Job drawing, mm, ordinate dimensions from the low corner. One solid piece. A direction names the side the tool comes from. Give positions to 0.01 mm unless a question says otherwise; leave off trailing zeros. Order: outer loops, then holes, each group sorted by start corner. A loop starts at its lowest first (then second) coordinate and runs counter-clockwise, first axis right, second up.
1. Which spindle directions (+Z, -Z, +X, -X, +Y, -Y) get a long thin tool onto all of the face, cutting with end or side? Do the marked faces 1, 2 and 3. Say none if no direction does.
2. Slice it at A-A on y = 12.7. List the corners of the cut face in (x, z), and give its area (3 significant figures).
3. Slice it at D-D on x = 190.5. List the corners of the cut face in (y, z).
4. Drop flat-ended pins along their axis: pin 1 Ø7.5 at (y, z) = (56, 10.5) entering from +X; pin 2 Ø10 at (x, z) = (234.5, 10) entering from +Y. Give the stop position or say it passes through.
5. Slice it at B-B on x = 279.4. List the corners of the cut face in (y, z).
6. Slice it at C-C on y = 63.5. List the corners of the cut face in (x, z).
7. Probe line 1 (Y direction, x = 114.3, z = 17.25); line 2 (X direction, y = 22, z = 11.5) (1 decimal); line 3 (X direction, y = 61, z = 5). List the from-to ranges inside material, lowest first.
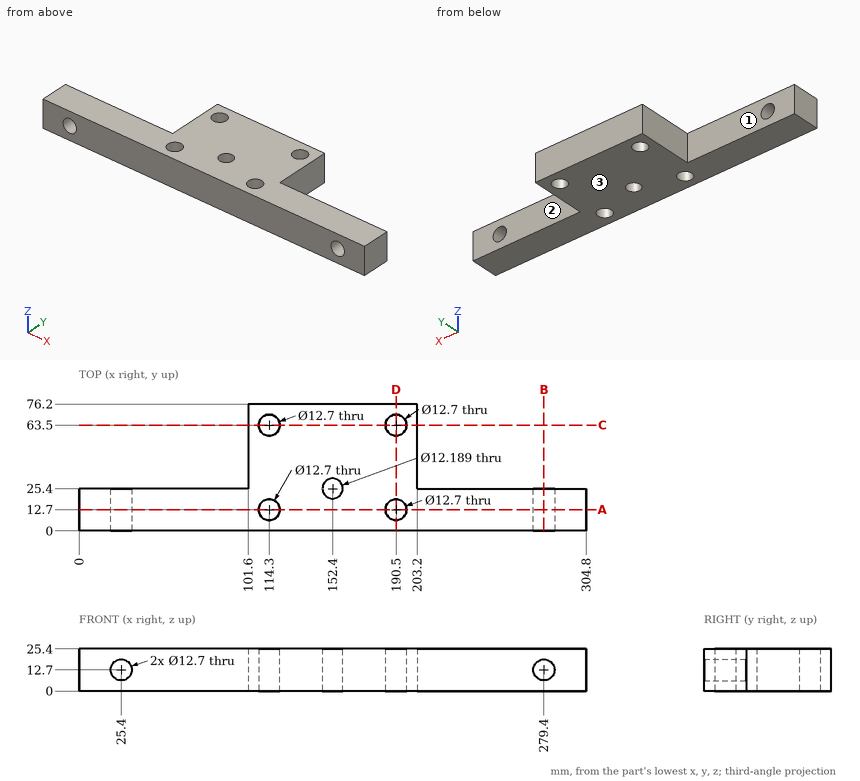
Data:
1. face 1: +Z, -Z, -X, +Y
1. face 2: +Z, -Z, +X, +Y
1. face 3: -Z, +X, -X, +Y, -Y
2. outline: (0, 0) - (107.95, 0) - (107.95, 25.4) - (0, 25.4) - close; (120.65, 0) - (184.15, 0) - (184.15, 25.4) - (120.65, 25.4) - close; (196.85, 0) - (304.8, 0) - (304.8, 25.4) - (196.85, 25.4) - close; hole circle Ø12.7 at (25.4, 12.7); hole circle Ø12.7 at (279.4, 12.7)
2. area: 6,840 mm2
3. outline: (0, 0) - (6.35, 0) - (6.35, 25.4) - (0, 25.4) - close; (19.05, 0) - (57.15, 0) - (57.15, 25.4) - (19.05, 25.4) - close; (69.85, 0) - (76.2, 0) - (76.2, 25.4) - (69.85, 25.4) - close
4. pin 1: stops at x = 203.2
4. pin 2: stops at y = 25.4
5. outline: (0, 0) - (25.4, 0) - (25.4, 6.35) - (0, 6.35) - close; (0, 19.05) - (25.4, 19.05) - (25.4, 25.4) - (0, 25.4) - close
6. outline: (101.6, 0) - (107.95, 0) - (107.95, 25.4) - (101.6, 25.4) - close; (120.65, 0) - (184.15, 0) - (184.15, 25.4) - (120.65, 25.4) - close; (196.85, 0) - (203.2, 0) - (203.2, 25.4) - (196.85, 25.4) - close
7. line 1: y = 0 to 6.35, 19.05 to 57.15, 69.85 to 76.2
7. line 2: x = 0 to 19.2, 31.6 to 147.3, 157.5 to 273.2, 285.6 to 304.8
7. line 3: x = 101.6 to 108.46, 120.14 to 184.66, 196.34 to 203.2
